from build123d import *

# Parameters (mm, degrees)
SALIENTE_EXTRUIR1_DEPTH    = 3
SALIENTE_EXTRUIR2_DEPTH    = 3
VACIADO1_T                 = -2
CROQUIS2_R                 = 2.1
CROQUIS2_R_2               = 4.5
AGUJEROS_FRONTALES_DEPTH   = 2.128355545
SALIENTE_EXTRUIR3_DEPTH    = 20
CORTAR_EXTRUIR2_DEPTH      = 140.049655499
CORTAR_EXTRUIR2_DEPTH_BACK = 140.049655499
CORTAR_EXTRUIR3_REACH      = 91.766
CROQUIS6_R                 = 1.65


with BuildPart() as part:
    # Croquis1 → Saliente-Extruir1 (new, along a direction that is not the sketch's normal)
    with BuildSketch(Plane.XY):
        with BuildLine():
            Line((51, 55.25), (-51, 55.25))
            ThreePointArc((-51, 55.25), (-58.071067812, 52.321067812), (-61, 45.25))
            Line((-61, 45.25), (-61, 38.85))
            Line((-61, 38.85), (-61, -45.25))
            ThreePointArc((-61, -45.25), (-58.071067812, -52.321067812), (-51, -55.25))
            Line((-51, -55.25), (51, -55.25))
            ThreePointArc((51, -55.25), (58.071067812, -52.321067812), (61, -45.25))
            Line((61, -45.25), (61, 38.85))
            Line((61, 38.85), (61, 45.25))
            ThreePointArc((61, 45.25), (58.071067812, 52.321067812), (51, 55.25))
        make_face()
        with BuildLine():
            ThreePointArc((-54.6, -38.85), (-51.671067812, -45.921067812), (-44.6, -48.85))
            Line((-44.6, -48.85), (44.6, -48.85))
            ThreePointArc((44.6, -48.85), (51.671067812, -45.921067812), (54.6, -38.85))
            Line((54.6, -38.85), (54.6, 33.85))
            Line((54.6, 33.85), (54.6, 38.85))
            ThreePointArc((54.6, 38.85), (51.671067812, 45.921067812), (44.6, 48.85))
            Line((44.6, 48.85), (-44.6, 48.85))
            ThreePointArc((-44.6, 48.85), (-51.671067812, 45.921067812), (-54.6, 38.85))
            Line((-54.6, 38.85), (-54.6, 33.85))
            Line((-54.6, 33.85), (-54.6, -38.85))
        make_face(mode=Mode.SUBTRACT)
        with BuildLine():
            Line((-54.6, 33.85), (-54.6, -38.85))
            ThreePointArc((-54.6, -38.85), (-51.671067812, -45.921067812), (-44.6, -48.85))
            Line((-44.6, -48.85), (44.6, -48.85))
            ThreePointArc((44.6, -48.85), (51.671067812, -45.921067812), (54.6, -38.85))
            Line((54.6, -38.85), (54.6, 33.85))
            Line((54.6, 33.85), (54.6, 38.85))
            ThreePointArc((54.6, 38.85), (51.671067812, 45.921067812), (44.6, 48.85))
            Line((44.6, 48.85), (-44.6, 48.85))
            ThreePointArc((-44.6, 48.85), (-51.671067812, 45.921067812), (-54.6, 38.85))
            Line((-54.6, 38.85), (-54.6, 33.85))
        make_face()
    extrude(amount=SALIENTE_EXTRUIR1_DEPTH, dir=(0, 0.34202014332566943, 0.9396926207859081))

    # Croquis1<3> → Saliente-Extruir2 (add, along a direction that is not the sketch's normal)
    with BuildSketch(Plane.XY):
        with BuildLine():
            Line((-54.6, 33.85), (-54.6, -38.85))
            ThreePointArc((-54.6, -38.85), (-51.671067812, -45.921067812), (-44.6, -48.85))
            Line((-44.6, -48.85), (44.6, -48.85))
            ThreePointArc((44.6, -48.85), (51.671067812, -45.921067812), (54.6, -38.85))
            Line((54.6, -38.85), (54.6, 33.85))
            Line((54.6, 33.85), (54.6, 38.85))
            ThreePointArc((54.6, 38.85), (51.671067812, 45.921067812), (44.6, 48.85))
            Line((44.6, 48.85), (-44.6, 48.85))
            ThreePointArc((-44.6, 48.85), (-51.671067812, 45.921067812), (-54.6, 38.85))
            Line((-54.6, 38.85), (-54.6, 33.85))
        make_face()
    extrude(amount=-SALIENTE_EXTRUIR2_DEPTH, dir=(0, 0.34202014332566943, 0.9396926207859081))

    # Vaciado1
    vaciado1_openings = [part.faces().sort_by_distance(p)[0] for p in [
        (0, -1.02606043, -2.819077862),
    ]]
    offset(amount=VACIADO1_T, openings=vaciado1_openings, kind=Kind.INTERSECTION)

    # Croquis2 → agujeros_frontales (cut, along a direction that is not the sketch's normal)
    with BuildSketch(Plane.XY.offset(2.819077862)):
        with Locations((1.522820459, 25.074336596)):
            Circle(CROQUIS2_R)
        with Locations((22.322818653, 8.874338039)):
            Circle(CROQUIS2_R)
        with Locations((22.422820346, -14.925662509)):
            Circle(CROQUIS2_R)
        with Locations((1.122821138, -32.425665611)):
            Circle(CROQUIS2_R)
        with Locations((-18.337182685, -15.02566234)):
            Circle(CROQUIS2_R)
        with Locations((-18.377177401, 9.074337699)):
            Circle(CROQUIS2_R)
        with Locations((1.910269276, 5.696006038)):
            Circle(CROQUIS2_R_2)
        with BuildLine():
            Line((-41.5, -28.97393957), (-41.5, 31.02606043))
            ThreePointArc((-41.5, 31.02606043), (-40, 32.52606043), (-38.5, 31.02606043))
            Line((-38.5, 31.02606043), (-38.5, -28.97393957))
            ThreePointArc((-38.5, -28.97393957), (-40, -30.47393957), (-41.5, -28.97393957))
        make_face()
        with BuildLine():
            Line((-32.5, -28.97393957), (-32.5, 31.02606043))
            ThreePointArc((-32.5, 31.02606043), (-34, 32.52606043), (-35.5, 31.02606043))
            Line((-35.5, 31.02606043), (-35.5, -28.97393957))
            ThreePointArc((-35.5, -28.97393957), (-34, -30.47393957), (-32.5, -28.97393957))
        make_face()
        with BuildLine():
            Line((41.5, -28.97393957), (41.5, 31.02606043))
            ThreePointArc((41.5, 31.02606043), (40, 32.52606043), (38.5, 31.02606043))
            Line((38.5, 31.02606043), (38.5, -28.97393957))
            ThreePointArc((38.5, -28.97393957), (40, -30.47393957), (41.5, -28.97393957))
        make_face()
        with BuildLine():
            Line((35.5, -28.97393957), (35.5, 31.02606043))
            ThreePointArc((35.5, 31.02606043), (34, 32.52606043), (32.5, 31.02606043))
            Line((32.5, 31.02606043), (32.5, -28.97393957))
            ThreePointArc((32.5, -28.97393957), (34, -30.47393957), (35.5, -28.97393957))
        make_face()
    extrude(amount=-AGUJEROS_FRONTALES_DEPTH, dir=(0, 0.34202014332566943, 0.9396926207859081), mode=Mode.SUBTRACT)

    # Croquis4 → Saliente-Extruir3 (add, along a direction that is not the sketch's normal)
    with BuildSketch(Plane.XY.offset(2.819077862)):
        with BuildLine():
            ThreePointArc((61, 46.27606043), (58.071067812, 53.347128242), (51, 56.27606043))
            Line((51, 56.27606043), (0, 56.27606043))
            Line((0, 56.27606043), (0, 54.27606043))
            Line((0, 54.27606043), (51, 54.27606043))
            ThreePointArc((51, 54.27606043), (56.656854249, 51.932914679), (59, 46.27606043))
            Line((59, 46.27606043), (59, -11.72393957))
            Line((59, -11.72393957), (61, -13.72393957))
            Line((61, -13.72393957), (61, 46.27606043))
        make_face()
        with BuildLine():
            Line((0, 54.27606043), (0, 56.27606043))
            Line((0, 56.27606043), (-51, 56.27606043))
            ThreePointArc((-51, 56.27606043), (-58.071067812, 53.347128242), (-61, 46.27606043))
            Line((-61, 46.27606043), (-61, -11.72393957))
            Line((-61, -11.72393957), (-61, -13.72393957))
            Line((-61, -13.72393957), (-59, -11.72393957))
            Line((-59, -11.72393957), (-59, 46.27606043))
            ThreePointArc((-59, 46.27606043), (-56.656854249, 51.932914679), (-51, 54.27606043))
            Line((-51, 54.27606043), (0, 54.27606043))
        make_face()
    extrude(amount=SALIENTE_EXTRUIR3_DEPTH, dir=(0, 0.3420201433256695, 0.9396926207859082))

    # Croquis5 → Cortar-Extruir2 (cut, two sides)
    with BuildSketch(Plane(origin=(61, 0, 0), x_dir=(0, 0, -1), z_dir=(1, 0, 0))) as cortar_extruir2_sk:
        with BuildLine():
            Line((-21.612930278, 53.116463296), (-21.612930278, -13.72393957))
            Line((-21.612930278, -13.72393957), (-2.819077862, -13.72393957))
            add(Edge.make_bspline(
                [(-21.612930278, 53.116463296), (-18.192805265, 26.402020841), (-24.202213901, 19.250300864), (-2.819077862, -13.72393957)],
                knots=[0.10784476, 0.10784476, 0.10784476, 0.10784476, 1, 1, 1, 1], degree=3))
        make_face()
    extrude(amount=CORTAR_EXTRUIR2_DEPTH, mode=Mode.SUBTRACT)
    extrude(cortar_extruir2_sk.sketch, amount=-CORTAR_EXTRUIR2_DEPTH_BACK, mode=Mode.SUBTRACT)

    # Croquis6 → Cortar-Extruir3 (cut, up to next)
    with BuildSketch(Plane.XY.offset(2.819077862), mode=Mode.PRIVATE) as cortar_extruir3_sk1:
        with Locations((0, -51.22393957)):
            Circle(CROQUIS6_R)
    cortar_extruir3_tool1 = extrude(cortar_extruir3_sk1.sketch, amount=-CORTAR_EXTRUIR3_REACH, mode=Mode.PRIVATE) & part.part
    add(cortar_extruir3_tool1.solids().sort_by_distance((0, -51.22394, 2.819078))[0], mode=Mode.SUBTRACT)


solid = part.part
For this review, take the finished solid that the model builds, in its own axes (mm). A direction names the side the tool comes from. Give positions to 0.01 mm unless a question says otherwise; leave off trailing zeros. Loops run counter-clockwise (first coordinate to the right, second up) from the corner with the lowest first, then second, coordinate; pieces in that order, holes last. Notation, with made-up numbers: M 35.5,30.25 L 65.5,30.25 A27 cw 65.5,50.25 Z; hole C 16,-30 d1. An arc over 180 degrees is marked long. Put each result on its own line as item: value. Start each with the question number.
(1) Wall thickness on L1, parallel to X at y = 50, z = 15; L2, parallel to Y at x = 0, z = 1; L3, parallel to Y at x = 0, z = 0.95: over which ranges is each line inside the solid? List them lowest first.
(2) The part is to be moulded in two halves that separate along Y. For faces 1 (the flat face through (0.62, 46.37, -0.97)), 2 (the flat face through (52.6, -1, -1)), 3 (the flat face through (0.71, 59.13, 10.66)), 4 (the flat face through (-53, -1, -2.819)), say which applies: +Y half, -Y half, draft (parallel to the pull), parting line (faces both ways), or undercut.
(3) Machinability: for faces 5 (the flat face through (-0.624, -47.076, -0.975)), 6 (the cylindrical face through (0.887, -49.833, 1.429)), 7 (the flat face through (-54.6, 0, -1)), 8 (the flat face through (59, 21, 10)), which of the approach directions +Z, -Z, +X, -X, +Y, -Y give a long, thin tool a straight path to every point of the face, cutting with its end or side? Answer none if there is none.
(4) For pin 1 (6 mm diameter, centred on x = 3.5, y = 18.5, fed in from -Z); pin 2 (6 mm diameter, centred on x = -38, z = 2.5, fed in from +Y); pin 3 (4 mm diameter, centred on x = -18.5, y = -7, fed in from +Z), all flat-tipped, find the tip position at first contact; note any pin that passes through.
(5) Add section A-A, the plane x = 15.5. Write out the cut boundary in (y, z).
Result:
1. L1: x = -61 to -59, 59 to 61
1. L2: y = -54.89 to -52.87, -49.57 to -34.86, -31.31 to 0.96, 9.11 to 22.97, 25.86 to 55.61
1. L3: y = -54.9 to -52.87, -49.57 to -34.88, -31.33 to 0.94, 9.09 to 22.95, 25.84 to 55.6
2. face 1: undercut
2. face 2: undercut
2. face 3: +Y half
2. face 4: draft
3. face 5: -Z
3. face 6: +Z
3. face 7: -Z, -X, +Y, -Y
3. face 8: +Z, -Y
4. pin 1: stops at z = 0.82
4. pin 2: stops at y = 57.25
4. pin 3: stops at z = 2.82
5. outline: M -55.25,0 L -48.85,0 L -49.88,-2.82 L -47.75,-2.82 L -46.42,0.82 L 47.02,0.82 L 45.7,-2.82 L 47.82,-2.82 L 48.85,0 L 55.25,0 L 63.12,21.61 L 61.12,21.61 L 54.28,2.82 L -54.22,2.82 Z
